The listing builds one solid part. Answer for the finished solid, in the listing's coordinates (mm). A direction names the side the tool comes from. Give positions to 0.01 mm unless a question says otherwise; leave off trailing zeros. Write each loop counter-clockwise with the first axis right and the second up, starting at its lowest first coordinate (ties: lowest second). Pieces come first, ordered by that corner, then holes. Notation, with made-up numbers: (-28.5, 46.25) - (27.5, 46.25) arc R11 ccw to (27.5, 63.25) - close; hole circle Ø7 at (84, 35.25). An arc over 180 degrees is marked (long way). Answer in a Markdown table with one row per item. Add a question column.
from build123d import *

# Parameters (mm, degrees)
BOSS_EXTRUDE1_DEPTH = 7.5
SKETCH2_R           = 5.25
CUT_EXTRUDE1_DEPTH  = 6
SKETCH4_R           = 2.75
CUT_EXTRUDE3_DEPTH  = 28
CUT_EXTRUDE4_REACH  = 36.369
SKETCH5_W           = 8
SKETCH5_H           = 5.1
CHAMFER2_SIZE       = 5
CHAMFER2_SIZE2      = 8.660254038
CHAMFER3_SIZE       = 4


with BuildPart() as part:
    # Sketch1 → Boss-Extrude1 (new, symmetric)
    with BuildSketch(Plane.XY):
        Polygon((-6, 8), (4, 8), (4, -30), (-11, -30), (-11, 0), (-1, 0), (-1, 4), (-6, 4), align=None)
    extrude(amount=BOSS_EXTRUDE1_DEPTH, both=True)

    # Sketch2 → Cut-Extrude1 (cut)
    with BuildSketch(Plane.XZ.offset(30)):
        with Locations((-3.5, 0)):
            Circle(SKETCH2_R)
    extrude(amount=-CUT_EXTRUDE1_DEPTH, mode=Mode.SUBTRACT)

    # Sketch4 → Cut-Extrude3 (cut)
    with BuildSketch(Plane.XZ.offset(30)):
        with Locations((-3.5, 0)):
            Circle(SKETCH4_R)
    extrude(amount=-CUT_EXTRUDE3_DEPTH, mode=Mode.SUBTRACT)

    # Sketch5 → Cut-Extrude4 (cut, up to next)
    with BuildSketch(Plane(origin=(4, 0, 0), x_dir=(0, 0, -1), z_dir=(1, 0, 0)), mode=Mode.PRIVATE) as cut_extrude4_sk1:
        with Locations((0, -16.55)):
            Rectangle(SKETCH5_W, SKETCH5_H)
    cut_extrude4_tool1 = extrude(cut_extrude4_sk1.sketch, amount=-CUT_EXTRUDE4_REACH, mode=Mode.PRIVATE) & part.part
    add(cut_extrude4_tool1.solids().sort_by_distance((4, -16.55, 0))[0], mode=Mode.SUBTRACT)

    # Chamfer2
    chamfer2_edges = [part.edges().sort_by_distance(p)[0] for p in [
        (-11, 0, 0),
    ]]
    chamfer2_side = [part.faces().sort_by_distance(p)[0] for p in [
        (-6, 0, 0),
    ]]
    chamfer(chamfer2_edges, length=CHAMFER2_SIZE, length2=CHAMFER2_SIZE2, reference=chamfer2_side[0])

    # Chamfer3
    # the kernel refuses this chamfer: 4 mm, written as the material it takes off along each edge
    with BuildSketch(Plane(origin=(-11, -40.286731952, 7.5), x_dir=(-0.027495876610586487, 0, -0.9996219169112968), z_dir=(0, 1, 0)), Plane(origin=(-11, -40.286731952, -7.5), x_dir=(0.9996219169112968, 0, -0.027495876610586275), z_dir=(0, 1, 0))) as chamfer3_piece_1:
        Polygon((CHAMFER3_SIZE * 0.999621916911, -CHAMFER3_SIZE * 0.0274958766106), (-CHAMFER3_SIZE * 0.0274958766106, -CHAMFER3_SIZE * 0.999621916911), (0, 0), align=None)
    extrude(amount=41.913209866, mode=Mode.SUBTRACT)
    with BuildSketch(Plane(origin=(4, 18.286731952, -7.5), x_dir=(-0.9996219169112968, 0, -0.027495876610586275), z_dir=(0, -1, 0)), Plane(origin=(4, 18.286731952, 7.5), x_dir=(0.02749587661058638, 0, -0.9996219169112968), z_dir=(0, -1, 0))) as chamfer3_piece_2:
        Polygon((CHAMFER3_SIZE * 0.999621916911, -CHAMFER3_SIZE * 0.0274958766106), (-CHAMFER3_SIZE * 0.0274958766106, -CHAMFER3_SIZE * 0.999621916911), (0, 0), align=None)
    extrude(amount=58.573463904, mode=Mode.SUBTRACT)


solid = part.part
1. Straight lines are drawn through the part: L1, parallel to Y at x = -2.75, z = 3.75; L2, parallel to Y at x = -4.5, z = 2; L3, parallel to Z at x = -3.5, y = -20.7. For each, find the intervals that lie inside material, in ascending order. Write a range as [from, to].
2. Given pin 1 Ø2.5 at (x, z) = (-3, 0.5) entering from -Y; pin 2 Ø4.5 at (y, z) = (2.5, -0.5) entering from -X; pin 3 Ø4 at (x, z) = (-1, -1) entering from -Y; pin 4 Ø5 at (y, z) = (-12, 4) entering from -X, each flat-ended and moving along its own axis, determine where each tip first touches the part or whether it passes through.
3. Section D-D (y = -16.5) is taken. Give the vertices of the cut face in (x, z).
4. Section B-B (x = -3.5) is taken. Give the vertices of the cut face in (y, z).
5. Section C-C (z = 0) is taken. Give the vertices of the cut face in (x, y).
6. The mould has two halves that part along Y. Classify faces 6 (the face through (-1, 2, 0)), 7 (the face through (2, -10.7, 5.5)), 8 (the face through (-1.7, -30, 5.1)), 9 (the face through (-5, -14, 3)): +Y half, -Y half, draft (parallel to the pull), parting line (faces both ways), or undercut.
7. A tool of negligible diameter and unlimited length cuts with its end or side. For faces 1 (the face through (-4, -2, 0)), 2 (the face through (-3, -17, 4)), 3 (the face through (-9, -19.2, 5.5)), 4 (the face through (4, -24, 0)), 5 (the face through (-3, 4, 0)), from which of +Z, -Z, +X, -X, +Y, -Y can it reach the whole face along a straight path? Write none if from no direction.
8. Section A-A (y = -26) is taken. Give the vertices of the cut face in (x, z).
Geometry check:
| question | item | result |
|---|---|---|
| 1 | L1 | [-24, -19.1], [-14, 0], [4, 8] |
| 1 | L2 | [-2, 0], [4, 8] |
| 1 | L3 | [-7.5, -2.75], [2.75, 7.5] |
| 2 | pin 1 | y = -2 |
| 2 | pin 2 | x = -6 |
| 2 | pin 3 | y = -24 |
| 2 | pin 4 | x = -11 |
| 3 | outline | (-10.5, -4) - (-7, -7.5) - (0, -7.5) - (3.5, -4) - close; (-10.5, 4) - (3.5, 4) - (0, 7.5) - (-7, 7.5) - close |
| 4 | outline | (-30, -7.5) - (0, -7.5) - (0, 7.5) - (-30, 7.5) - (-30, 5.25) - (-24, 5.25) - (-24, 2.75) - (-19.1, 2.75) - (-19.1, 4) - (-14, 4) - (-14, 2.75) - (-2, 2.75) - (-2, -2.75) - (-14, -2.75) - (-14, -4) - (-19.1, -4) - (-19.1, -2.75) - (-24, -2.75) - (-24, -5.25) - (-30, -5.25) - close; (4, -7.5) - (8, -7.5) - (8, 7.5) - (4, 7.5) - close |
| 5 | outline | (-11, -30) - (-8.75, -30) - (-8.75, -24) - (-6.25, -24) - (-6.25, -19.1) - (-11, -19.1) - close; (-11, -14) - (-6.25, -14) - (-6.25, -2) - (-0.75, -2) - (-0.75, -14) - (4, -14) - (4, 8) - (-6, 8) - (-6, 4) - (-1, 4) - (-1, 0) - (-6, 0) - (-11, -8.66) - close; (-0.75, -24) - (1.75, -24) - (1.75, -30) - (4, -30) - (4, -19.1) - (-0.75, -19.1) - close |
| 6 | face 6 | undercut |
| 6 | face 7 | draft |
| 6 | face 8 | -Y half |
| 6 | face 9 | undercut |
| 7 | face 1 | -Y |
| 7 | face 2 | +X, -X |
| 7 | face 3 | +Z, -X, +Y, -Y |
| 7 | face 4 | +Z, -Z, +X, +Y, -Y |
| 7 | face 5 | +Z, -Z, -X |
| 8 | outline | (-11, -3.5) - (-7, -7.5) - (0, -7.5) - (4, -3.5) - (4, 3.5) - (0, 7.5) - (-7, 7.5) - (-11, 3.5) - close; hole circle Ø10.5 at (-3.5, 0) |
